```python
from build123d import *

# Parameters (mm, degrees)
PAD_DEPTH    = 9
SKETCH001_R  = 1.5
POCKET_DEPTH = 9.001


with BuildPart() as part:
    # Sketch → Pad (new body)
    with BuildSketch(Plane.XY):
        Polygon((0, 0), (0, 120), (120, 0), align=None)
    extrude(amount=-PAD_DEPTH)

    # Sketch001 (on Face4 of Pad) → Pocket (cut, through all)
    with BuildSketch(Plane.XY):
        with Locations((5, 30)):
            Circle(SKETCH001_R)
        with Locations((5, 90)):
            Circle(SKETCH001_R)
        with Locations((30, 5)):
            Circle(SKETCH001_R)
        with Locations((90, 5)):
            Circle(SKETCH001_R)
    extrude(amount=-POCKET_DEPTH, mode=Mode.SUBTRACT)


solid = part.part
```
The model under review builds one solid part; all positions refer to its coordinate system, in mm. Give positions to 0.01 mm unless a question says otherwise; leave off trailing zeros. Write each loop counter-clockwise with the first axis right and the second up, starting at its lowest first coordinate (ties: lowest second). Pieces come first, ordered by that corner, then holes. Notation, with made-up numbers: M 89.25,6.5 L 110.25,6.5 A24 ccw 110.25,34.5 Z; hole C 21,-13.5 d10. An arc over 180 degrees is marked long. Write item = value, one per line. Start each with the question number.
Q1. Mouldability with a two-part tool opening along X and no side actions: class faces 1 (the face through (4.805, 91.487, -4.437)), 2 (the face through (0, 59, -4)), 3 (the face through (61, 0, -4)) as released by +X, released by -X, zero draft, split by the parting line, or undercut.
Q2. For line 1 (Y direction, x = 5, z = -7); line 2 (Y direction, x = 30, z = -2.25); line 3 (X direction, y = 90, z = -5.75), list the stretches that pass through material, from the lowest coordinate up.
Q3. We need section C-C (z = -5.25). State the section outline as (x, y) points.
Q4. We need section B-B (x = 30). State the section outline as (y, z) points, plus the area to 3 significant figures.
Q5. We need section D-D (x = 107.5). State the section outline as (y, z) points.
Q6. Clearance check with flat-ended pins moving along their axes: pin 1 (2 mm diameter, centred on x = 36.5, z = -4.5, fed in from -Y); pin 2 (2.5 mm diameter, centred on x = 30, y = 5, fed in from +Z). State where each tip first meets the part, or that it passes through.
Q7. We need section A-A (y = 90). State the section outline as (x, z) points.
Result set:
q1.face_1 = undercut
q1.face_2 = released by -X
q1.face_3 = zero draft
q2.line_1 = 0 to 28.5, 31.5 to 88.5, 91.5 to 115
q2.line_2 = 0 to 3.5, 6.5 to 90
q2.line_3 = 0 to 3.5, 6.5 to 30
q3.outline = M 0,0 L 120,0 L 0,120 Z; hole C 5,30 d3; hole C 5,90 d3; hole C 30,5 d3; hole C 90,5 d3
q4.outline = M 0,-9 L 3.5,-9 L 3.5,0 L 0,0 Z; M 6.5,-9 L 90,-9 L 90,0 L 6.5,0 Z
q4.area = 783 mm2
q5.outline = M 0,-9 L 12.5,-9 L 12.5,0 L 0,0 Z
q6.pin_1 = 0
q6.pin_2 = through
q7.outline = M 0,-9 L 3.5,-9 L 3.5,0 L 0,0 Z; M 6.5,-9 L 30,-9 L 30,0 L 6.5,0 Z
